Verification items for this drawing (mm, ordinates from the low corner). Round coordinates to 2 decimals unless told otherwise and drop trailing zeros. Order: outer loops, then holes, each group sorted by start corner. A loop starts at its lowest first (then second) coordinate and runs counter-clockwise, first axis right, second up.
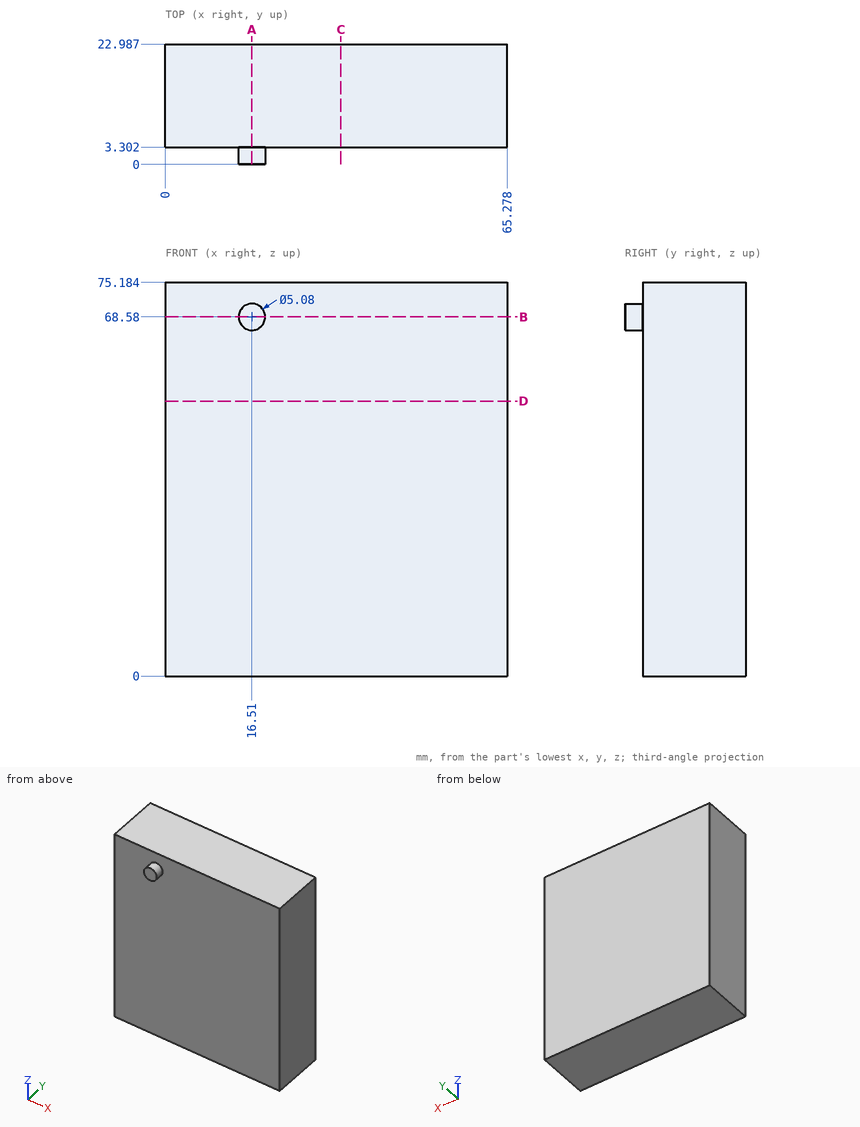
Item 1: Sectioned sample at C-C (x = 33.5). Record the cut outline in (y, z).
Answer:
outline: (3.3, 0) - (22.99, 0) - (22.99, 75.18) - (3.3, 75.18) - close
Item 2: Sectioned sample at D-D (z = 52.5). Record the cut outline in (x, y), and give its area (4 significant figures).
Answer:
outline: (0, 3.3) - (65.28, 3.3) - (65.28, 22.99) - (0, 22.99) - close
area: 1,285 mm2
Item 3: Sectioned sample at B-B (z = 68.58). Record the cut outline in (x, y), and give its area (3 significant figures).
Answer:
outline: (0, 3.3) - (13.97, 3.3) - (13.97, 0) - (19.05, 0) - (19.05, 3.3) - (65.28, 3.3) - (65.28, 22.99) - (0, 22.99) - close
area: 1,300 mm2
Item 4: Go/stop test with flat-tipped pins: P1, Ø5, axis at y = 2.5, z = 28, coming from the -X side; P2, Ø4, axis at x = 47, z = 20.5, coming from the -Y side. Record where each tip stops, or that it passes through.
Answer:
P1: stops at x = 0
P2: stops at y = 3.3
Item 5: Scan line: line 1 along Y through (x, z) = (18, 63). Record every from-to range of solid material in increasing order.
Answer:
line 1: y = 3.3 to 22.99
Item 6: Sectioned sample at A-A (x = 16.51). Record the cut outline in (y, z), and give its area (3 significant figures).
Answer:
outline: (0, 66.04) - (3.3, 66.04) - (3.3, 0) - (22.99, 0) - (22.99, 75.18) - (3.3, 75.18) - (3.3, 71.12) - (0, 71.12) - close
area: 1,500 mm2
